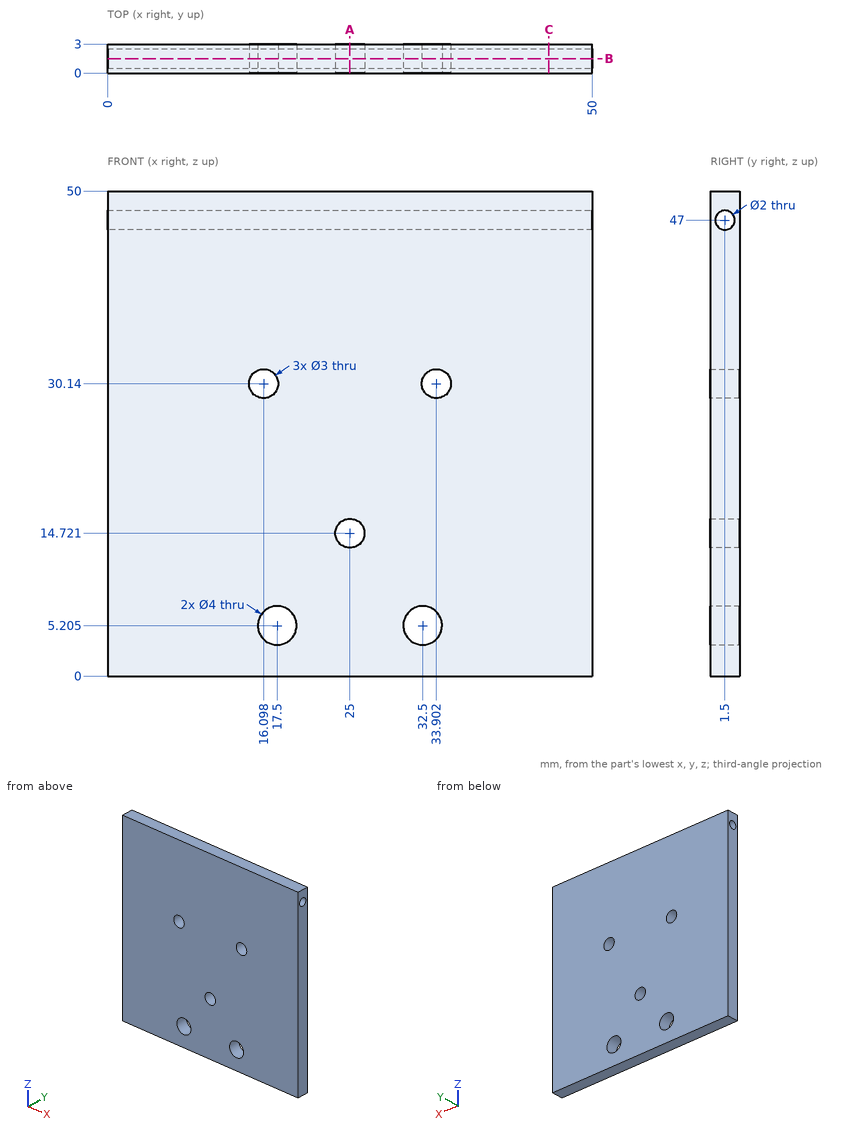
The figure shows three views and two pictorial views of one solid part (mm, origin at its lowest corner). Answer the questions. Give positions to 0.01 mm unless a question says otherwise; leave off trailing zeros. Write each loop counter-clockwise with the first axis right and the second up, starting at its lowest first coordinate (ties: lowest second). Pieces come first, ordered by that corner, then holes. Notation, with made-up numbers: (-17.5, 73.25) - (16.5, 73.25) arc R18 cw to (16.5, 93.25) - close; hole circle Ø3 at (74, 82). An arc over 180 degrees is marked (long way). Use one line per item in the form item = value. Start each with the question number.
1) Consider line 1 along X through (y, z) = (2.45, 30) (1 decimal); line 2 along Y through (x, z) = (40, 47); line 3 along Z through (x, y) = (32, 1.4) (1 decimal). Determine where each line is inside the solid, lowest interval first. Write a range as from..to.
2) Find section B-B on y = 1.5. Determine the outline of the cut face in (x, z) (1 decimal).
3) A flat-ended cylindrical pin translates along its axis: pin 1 Ø2.5 at (x, z) = (17.5, 5.21) entering from +Y. Find the tip coordinate at first contact, or state that the pin passes through.
4) Find section C-C on x = 45.5. Determine the outline of the cut face in (y, z).
5) Find section A-A on x = 25. Determine the outline of the cut face in (y, z), plus the area to 3 significant figures.
Geometry results:
q1.line_1 = 0..14.6, 17.6..32.4, 35.4..50
q1.line_2 = 0..0.5, 2.5..3
q1.line_3 = 0..3.3, 7.1..46, 48..50
q2.outline = (0, 0) - (50, 0) - (50, 46) - (0, 46) - close; (0, 48) - (50, 48) - (50, 50) - (0, 50) - close; hole circle Ø3 at (16.1, 30.1); hole circle Ø4 at (17.5, 5.2); hole circle Ø3 at (25, 14.7); hole circle Ø4 at (32.5, 5.2); hole circle Ø3 at (33.9, 30.1)
q3.pin_1 = through
q4.outline = (0, 0) - (3, 0) - (3, 50) - (0, 50) - close; hole circle Ø2 at (1.5, 47)
q5.outline = (0, 0) - (3, 0) - (3, 13.22) - (0, 13.22) - close; (0, 16.22) - (3, 16.22) - (3, 50) - (0, 50) - close; hole circle Ø2 at (1.5, 47)
q5.area = 138 mm2
